Autodesk Inventor part; units mm, degrees
ref_plane "YZ Plane" through (0, 0, 0) normal (1, 0, 0) x (0, 1, 0)
ref_plane "XZ Plane" through (0, 0, 0) normal (0, 1, 0) x (-1, 0, 0)
ref_plane "XY Plane" through (0, 0, 0) normal (0, 0, 1) x (1, 0, 0)
sketch "Sketch1" plane through (0, 0, 0) normal (0, 0, 1) x (1, 0, 0)
  line L0 (0, 0) -> (0, 2.5)
  line L1 (0, 2.5) -> (-2.2441, 7.6403)
  line L2 (-2.2441, 7.6403) -> (4.9187, 10.7674)
  line L3 (4.9187, 10.7674) -> (7, 6)
  line L4 (7, 6) -> (7, 0)
  line L5 (7, 0) -> (0, 0)
  dimension "d5" = 23.584
  dimension "d6" = 2.5
  dimension "d7" = 7
  dimension "d9" = 6
  dimension "d14" = 7.9
extrude "Extrusion1" add sketch "Sketch1" along normal blind 10
sketch "Sketch2" plane through (6.9048, 6.218, 0) normal (-0.916472, -0.4000988, 0) x (0, 0, 1)
  line L0 (0, 4.964) -> (10, 4.964)
  line L1 (10, 4.964) -> (10, -0.6448)
  line L2 (10, 4.964) -> (0, 1.618)
  line L3 (0, 1.618) -> (0, 4.964)
  point P0 (0, -2.936)
  dimension "d2" = 18.5
extrude "Extrusion2" cut sketch "Sketch2" along normal through all both and the other way through all
sketch "Sketch3" plane through (0, 0, 0) normal (0, -1, 0) x (1, 0, 0)
  line L0 (7, 0) -> (0, 0)
  line L1 (7, 0) -> (7, 10)
  line L2 (0, 10) -> (7, 10)
  line L3 (0, 0) -> (0, 10)
  line L4 (2.5, 10) -> (7, 0.5)
  dimension "d12" = 2.5
  dimension "d13" = 0.5
extrude "Extrusion3" cut sketch "Sketch3" against normal through all contours L4 L2 L1
sketch "Sketch4" plane through (0, 0, 0) normal (0, -1, 0) x (1, 0, 0)
  point P0 (0, 0)
  point P1 (3, 2)
  point P2 (1.8, 7)
  dimension "d22" = 3
  dimension "d23" = 2
  dimension "d24" = 7
  dimension "d25" = 1.8
hole "Hole1" at (3, 0, 2) at (1.8, 0, 7) direction (0, 1, 0) diameter 1.567 depth 5 tip angle 118
equation "\"d5\" = thumb_axis_beta_local"
equation "\"thumb_axis_beta_local\" = thumb_axis_beta"
properties part number "CMC extension endstop"
Can you work these out from the model? Positions are in its coordinate system, mm. A direction names the side the tool comes from. Give positions to 0.01 mm unless a question says otherwise; leave off trailing zeros. Write each loop counter-clockwise with the first axis right and the second up, starting at its lowest first coordinate (ties: lowest second). Pieces come first, ordered by that corner, then holes. Notation, with made-up numbers: (-8.75, 30.5) -> (20.25, 30.5) arc R22 cw to (20.25, 62.5) -> close; hole circle Ø1 at (23.25, 52). An arc over 180 degrees is marked (long way). One line per item, written item: value.
Q1. Which directions (+Z, -Z, +X, -X, +Y, -Y) give clear straight access to the entire face, cutting with the end or side of a thin tool? Please do faces 4 (the face through (0, 1, 5)), 5 (the face through (3.695, 2.535, 1.638)), 6 (the face through (4.718, 4.788, 5.317)).
Results found:
face 4: +Z, -Z, -X, -Y
face 5: -Y
face 6: +Z, +X, +Y, -Y
Q2. Imagine slicing it at B-B on z = 8.5. Please give me the cut outline in (x, y), and give its area (3 significant figures).
Results found:
outline: (-2.04, 7.18) -> (0, 2.5) -> (0, 0) -> (3.21, 0) -> (3.21, 9.47) -> close
area: 33.9 mm^2
Q3. Imagine slicing it at A-A on y = 4.25. Please give me the cut outline in (x, z), and give its area (3 significant figures).
Results found:
outline: (-0.76, 0) -> (7, 0) -> (7, 0.5) -> (2.5, 10) -> (-0.76, 10) -> close; hole circle Ø1.57 at (1.8, 7); hole circle Ø1.57 at (3, 2)
area: 52.4 mm^2
Q4. Imagine slicing it at C-C on x = 0.5. Please give me the cut outline in (y, z).
Results found:
outline: (0, 0) -> (5.19, 0) -> (8.84, 10) -> (0, 10) -> close
Q5. We'd pull the mould along Z, two halves only. Please class faces 1 (the face through (6.43, 7.31, 1.1)), 2 (the face through (1, 5, 10)), 3 (the face through (1.14, 2.54, 6.58)): +Z half, -Z half, draft (parallel to the pull), parting line (faces both ways), or undercut.
Results found:
face 1: draft
face 2: +Z half
face 3: undercut
Q6. Please list where these lines run through material, in increasing order: line 1 (Z direction, x = 1.8, y = 2.25); line 2 (Z direction, x = 3.25, y = 4.25); line 3 (X direction, y = 2.2, z = 7). Write a range as [from, to].
Results found:
line 1: z = [0, 6.22], [7.78, 10]
line 2: z = [0, 1.26], [2.74, 8.42]
line 3: x = [0, 1.02], [2.58, 3.92]
Q7. For P1, Ø0.8, axis at y = 1.5, z = 3, coming from the -X side; P2, Ø1.3, axis at x = 1.8, z = 7, coming from the +Y side; P3, Ø2, axis at y = 5, z = 3, coming from the +X side, each with a flat end and sliding along its axis, tell me the tip position at first contact or that it passes through.
Results found:
P1: stops at x = 0
P2: stops at y = 8.68
P3: stops at x = 6.29
Q8. Imagine slicing it at D-D on y = 6.5. Please give me the cut outline in (x, z), and give its area (3 significant figures).
Results found:
outline: (-1.75, 6.28) -> (3.51, 0) -> (6.78, 0) -> (6.78, 0.96) -> (2.5, 10) -> (-1.75, 10) -> close
area: 49.4 mm^2
